from build123d import *

# Parameters (mm, degrees)
SM_BASE_FLANGE_1_DEPTH         = 123
SKETCH_2_W                     = 6
SKETCH_2_H                     = 12
CUT_EXTRUDE_1_DEPTH            = 1
SKETCH_3_W                     = 9.5
SKETCH_3_H                     = 4.5
CUT_EXTRUDE_2_DEPTH            = 1
FILLET_1_R                     = 2.25
SKETCH_4_R                     = 2.25
CUT_EXTRUDE_3_DEPTH            = 1
PATTERN_LINEAR_1_COUNT         = 2
PATTERN_LINEAR_1_PITCH         = 109.7
FILLET_1_OF_PATTERN_LINEAR_1_R = 2.25
PATTERN_LINEAR_2_COUNT         = 2
PATTERN_LINEAR_2_PITCH         = 188.2
FILLET_1_OF_PATTERN_LINEAR_2_R = 2.25
PATTERN_LINEAR_3_COUNT         = 2
PATTERN_LINEAR_3_PITCH         = 59.7
PATTERN_LINEAR_4_COUNT         = 2
PATTERN_LINEAR_4_PITCH         = 138.2


# Sheet-metal steps are written as plain solids
with BuildPart() as part:
    # Sketch 1 → Базовая кромка1 (new, symmetric)
    with BuildSketch(Plane.XY):
        with BuildLine():
            Line((6.5, 9.25), (1.2, 9.25))
            ThreePointArc((1.2, 9.25), (0.351471863, 8.898528137), (0, 8.05))
            Line((0, 8.05), (0, -8.05))
            ThreePointArc((0, -8.05), (0.351471863, -8.898528137), (1.2, -9.25))
            Line((1.2, -9.25), (6.5, -9.25))
            Line((6.5, -9.25), (6.5, -8.25))
            Line((6.5, -8.25), (1.2, -8.25))
            ThreePointArc((1.2, -8.25), (1.058578644, -8.191421356), (1, -8.05))
            Line((1, -8.05), (1, 8.05))
            ThreePointArc((1, 8.05), (1.058578644, 8.191421356), (1.2, 8.25))
            Line((1.2, 8.25), (6.5, 8.25))
            Line((6.5, 8.25), (6.5, 9.25))
        make_face()
    extrude(amount=SM_BASE_FLANGE_1_DEPTH, both=True)

    # Эскиз2 → Вытянуть1 (cut)
    with BuildSketch(Plane.ZY):
        with Locations((120, 0)):
            Rectangle(SKETCH_2_W, SKETCH_2_H)
    extrude(amount=-CUT_EXTRUDE_1_DEPTH, mode=Mode.SUBTRACT)

    # Эскиз3 → Вытянуть2 (cut)
    with BuildSketch(Plane.ZY):
        with Locations((94.25, 0)):
            Rectangle(SKETCH_3_W, SKETCH_3_H)
    cut_extrude_2 = extrude(amount=-CUT_EXTRUDE_2_DEPTH, mode=Mode.SUBTRACT)

    # Скругление1
    fillet_1_edges = [part.edges().sort_by_distance(p)[0] for p in [
        (0.5, 2.25, 99),
        (0.5, -2.25, 99),
        (0.5, 2.25, 89.5),
        (0.5, -2.25, 89.5),
    ]]
    fillet(fillet_1_edges, radius=FILLET_1_R - 0.0001)  # a hair under: the kernel refuses the full size

    # Эскиз4 → Вытянуть3 (cut)
    with BuildSketch(Plane.ZY):
        with Locations(Location((69.25, 0, 0), (0, 0, 270))):
            Circle(SKETCH_4_R)
    cut_extrude_3 = extrude(amount=-CUT_EXTRUDE_3_DEPTH, mode=Mode.SUBTRACT)

    # Линейный массив1: Вытянуть2 ×2
    with Locations(*[(0, 0, -i * PATTERN_LINEAR_1_PITCH) for i in range(1, PATTERN_LINEAR_1_COUNT)]):
        add(cut_extrude_2, mode=Mode.SUBTRACT)

    # Скругление1 of Линейный массив1
    fillet_1_of_pattern_linear_1_edges = [part.edges().sort_by_distance(p)[0] for p in [
        (0.5, 2.25, -10.7),
        (0.5, -2.25, -10.7),
        (0.5, 2.25, -20.2),
        (0.5, -2.25, -20.2),
    ]]
    fillet(fillet_1_of_pattern_linear_1_edges, radius=FILLET_1_OF_PATTERN_LINEAR_1_R - 0.0001)  # a hair under: the kernel refuses the full size

    # Линейный массив2: Вытянуть2 ×2
    with Locations(*[(0, 0, -i * PATTERN_LINEAR_2_PITCH) for i in range(1, PATTERN_LINEAR_2_COUNT)]):
        add(cut_extrude_2, mode=Mode.SUBTRACT)

    # Скругление1 of Линейный массив2
    fillet_1_of_pattern_linear_2_edges = [part.edges().sort_by_distance(p)[0] for p in [
        (0.5, 2.25, -89.2),
        (0.5, -2.25, -89.2),
        (0.5, 2.25, -98.7),
        (0.5, -2.25, -98.7),
    ]]
    fillet(fillet_1_of_pattern_linear_2_edges, radius=FILLET_1_OF_PATTERN_LINEAR_2_R - 0.0001)  # a hair under: the kernel refuses the full size

    # Линейный массив3: Вытянуть3 ×2
    with Locations(*[(0, 0, -i * PATTERN_LINEAR_3_PITCH) for i in range(1, PATTERN_LINEAR_3_COUNT)]):
        add(cut_extrude_3, mode=Mode.SUBTRACT)

    # Линейный массив4: Вытянуть3 ×2
    with Locations(*[(0, 0, -i * PATTERN_LINEAR_4_PITCH) for i in range(1, PATTERN_LINEAR_4_COUNT)]):
        add(cut_extrude_3, mode=Mode.SUBTRACT)


solid = part.part
Work out the finished part from the listing and answer in its coordinate system (mm). A direction names the side the tool comes from. Give positions to 0.01 mm unless a question says otherwise; leave off trailing zeros. Order: outer loops, then holes, each group sorted by start corner. A loop starts at its lowest first (then second) coordinate and runs counter-clockwise, first axis right, second up. Notation, with made-up numbers: (5.5, -6.75) -> (37.5, -6.75) arc R29 ccw to (37.5, 23.25) -> close; hole circle Ø10 at (-5, -17). An arc over 180 degrees is marked (long way). Answer as a JSON object with one key per item and string values. Group by question number.
1. A tool of negligible diameter and unlimited length cuts with its end or side. For faces 1 (the flat face through (4, 8.25, 2)), 2 (the flat face through (0.8, 1.4, -123)), from which of +Z, -Z, +X, -X, +Y, -Y can it reach the whole face along a straight path? Write none if from no direction.
2. Section A-A on z = -68.95 is taken. Determine the outline of the cut face in (x, y).
3. Flat-ended cylindrical pins translate along their axes: pin 1 Ø8 at (y, z) = (0, 15) entering from +X; pin 2 Ø1.1 at (x, z) = (0.5, -16) entering from +Y; pin 3 Ø0.5 at (x, z) = (0.5, 95.5) entering from -Y; pin 4 Ø4 at (y, z) = (-6.5, -13.5) entering from +X. Find the tip coordinate at first contact, or state that the pin passes through.
4. The mould has two halves that part along Y. Classify faces 3 (the flat face through (4, -9.25, 2)), 4 (the flat face through (1, 0, 2)), 5 (the flat face through (4, 9.25, 2)): released by +Y, released by -Y, zero draft, split by the parting line, or undercut.
5. Section B-B on x = 5.5 is taken. Determine the outline of the cut face in (y, z), plus the area to 3 significant figures.
6. Consider line 1 along Y through (x, z) = (3, -85.5); line 2 along X through (y, z) = (-6.5, -69.5); line 3 along Z through (x, y) = (0.5, -2.5). Determine where each line is inside the solid, lowest interval first. Write a range as [from, to].
7. Section C-C on z = -38.5 is taken. Determine the outline of the cut face in (x, y), plus the area to 3 significant figures.
Result sheet:
{
 "1": {"face 1": "+Z, -Z, +X", "face 2": "-Z, +X, -X, +Y, -Y"},
 "2": {"outline": "(0, -8.05) arc R1.2 ccw to (1.2, -9.25) -> (6.5, -9.25) -> (6.5, -8.25) -> (1.2, -8.25) arc R0.2 cw to (1, -8.05) -> (1, -2.25) -> (0, -2.25) -> close; (0, 2.25) -> (1, 2.25) -> (1, 8.05) arc R0.2 cw to (1.2, 8.25) -> (6.5, 8.25) -> (6.5, 9.25) -> (1.2, 9.25) arc R1.2 ccw to (0, 8.05) -> close"},
 "3": {"pin 1": "stops at x = 1", "pin 2": "stops at y = 9.24", "pin 3": "stops at y = -9.16", "pin 4": "stops at x = 6.5"},
 "4": {"face 3": "released by -Y", "face 4": "undercut", "face 5": "released by +Y"},
 "5": {"outline": "(-9.25, -123) -> (-8.25, -123) -> (-8.25, 123) -> (-9.25, 123) -> close; (8.25, -123) -> (9.25, -123) -> (9.25, 123) -> (8.25, 123) -> close", "area": "492 mm^2"},
 "6": {"line 1": "y = [-9.25, -8.25], [8.25, 9.25]", "line 2": "x = [0, 1]", "line 3": "z = [-123, 117]"},
 "7": {"outline": "(0, -8.05) arc R1.2 ccw to (1.2, -9.25) -> (6.5, -9.25) -> (6.5, -8.25) -> (1.2, -8.25) arc R0.2 cw to (1, -8.05) -> (1, 8.05) arc R0.2 cw to (1.2, 8.25) -> (6.5, 8.25) -> (6.5, 9.25) -> (1.2, 9.25) arc R1.2 ccw to (0, 8.05) -> close", "area": "28.9 mm^2"}
}
